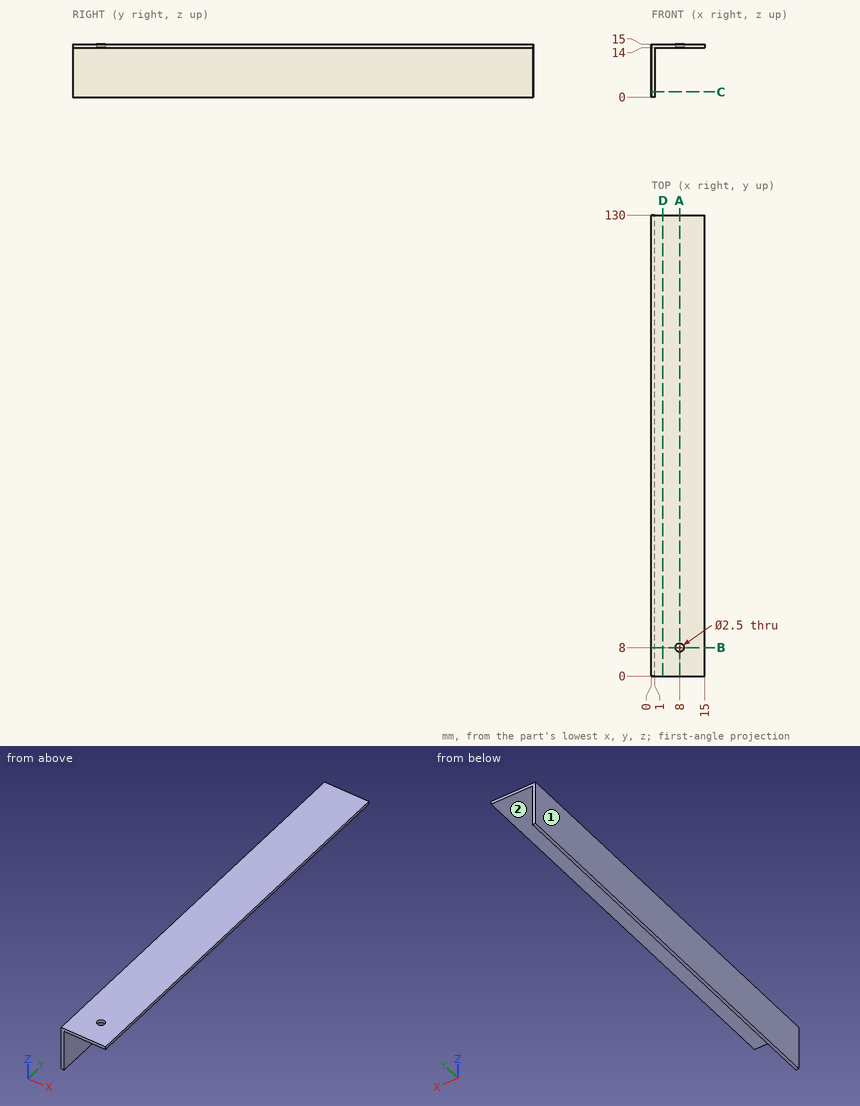
Can you work these out from the drawing? Everything is in mm from the part's minimum corner. A direction names the side the tool comes from. Give positions to 0.01 mm unless a question says otherwise; leave off trailing zeros. Order: outer loops, then holes, each group sorted by start corner. A loop starts at its lowest first (then second) coordinate and runs counter-clockwise, first axis right, second up. Notation, with made-up numbers: M 8,19 L 22,19 A28 ccw 22,38 Z; hole C -14,82.5 d8. An arc over 180 degrees is marked long. Write item = value, one per line. Start each with the question number.
Q1. Suppose I cut it at D-D (x = 3.25). Write out the boundary of the cut face in (y, z), plus the area to 3 significant figures.
Q2. Suppose I cut it at B-B (y = 8). Write out the boundary of the cut face in (x, z).
Q3. Suppose I cut it at C-C (z = 1.5). Write out the boundary of the cut face in (x, y), plus the area to 3 significant figures.
Q4. I need wall thicknesses on probe 1 along Y at (x, z) = (8, 14.2); probe 2 along X at (y, z) = (54, 4.25); probe 3 along Z at (x, y) = (10, 113). Which ranges of each line are inside material? Lowest first, please. Write a range as [from, to].
Q5. For the marked faces 1 and 2, which set-ups out of +Z, -Z, +X, -X, +Y, -Y let a thin tool reach every point of the face, with its end or its side?
Q6. Suppose I cut it at A-A (x = 8). Write out the boundary of the cut face in (y, z), plus the area to 4 significant figures.
Q7. Will these pins go through, and if not, where does the flat tip stop? pin 1 Ø1.5 at (y, z) = (111, 3.5) entering from +X; pin 2 Ø7 at (x, y) = (7, 67) entering from -Z; pin 3 Ø1 at (x, z) = (5, 12.5) entering from -Y.
Check result:
q1.outline = M 0,14 L 130,14 L 130,15 L 0,15 Z
q1.area = 130 mm2
q2.outline = M 0,0 L 1,0 L 1,14 L 6.75,14 L 6.75,15 L 0,15 Z; M 9.25,14 L 15,14 L 15,15 L 9.25,15 Z
q3.outline = M 0,0 L 1,0 L 1,130 L 0,130 Z
q3.area = 130 mm2
q4.probe_1 = [0, 6.75], [9.25, 130]
q4.probe_2 = [0, 1]
q4.probe_3 = [14, 15]
q5.face_1 = +Z, -Z, -X, +Y, -Y
q5.face_2 = -Z, +X, +Y, -Y
q6.outline = M 0,14 L 6.75,14 L 6.75,15 L 0,15 Z; M 9.25,14 L 130,14 L 130,15 L 9.25,15 Z
q6.area = 127.5 mm2
q7.pin_1 = 1
q7.pin_2 = 14
q7.pin_3 = through
